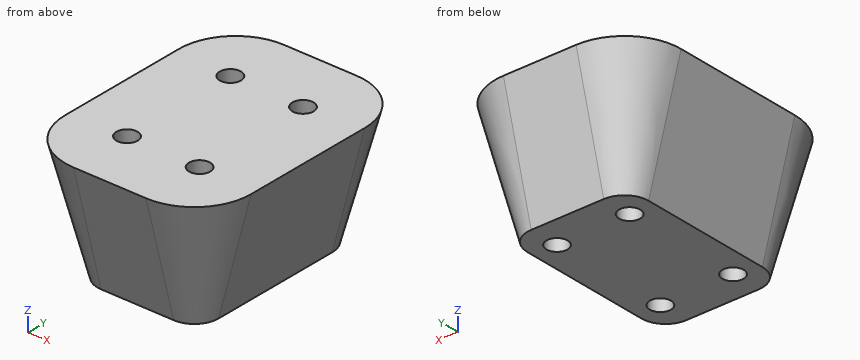
from build123d import *

# Parameters (mm, degrees)
SKETCH1_R           = 1.75
BOSS_EXTRUDE1_DEPTH = 5
BOSS_EXTRUDE2_DEPTH = 20
BOSS_EXTRUDE2_DRAFT = -15
CUT_EXTRUDE1_REACH  = 37.713
SKETCH5_R           = 1.75
CUT_EXTRUDE2_DEPTH  = 5


with BuildPart() as part:
    # Sketch1 → Boss-Extrude1 (new body)
    with BuildSketch(Plane.XY):
        with BuildLine():
            Line((-6, 15), (6, 15))
            ThreePointArc((6, 15), (8.828427125, 13.828427125), (10, 11))
            Line((10, 11), (10, -11))
            ThreePointArc((10, -11), (8.828427125, -13.828427125), (6, -15))
            Line((6, -15), (-6, -15))
            ThreePointArc((-6, -15), (-8.828427125, -13.828427125), (-10, -11))
            Line((-10, -11), (-10, 11))
            ThreePointArc((-10, 11), (-8.828427125, 13.828427125), (-6, 15))
        make_face()
        with Locations((-6, 10)):
            Circle(SKETCH1_R, mode=Mode.SUBTRACT)
        with Locations((6, 10)):
            Circle(SKETCH1_R, mode=Mode.SUBTRACT)
        with Locations((-6, -10)):
            Circle(SKETCH1_R, mode=Mode.SUBTRACT)
        with Locations((6, -10)):
            Circle(SKETCH1_R, mode=Mode.SUBTRACT)
    extrude(amount=BOSS_EXTRUDE1_DEPTH)


with BuildPart() as boss_extrude2_tool:
    # Sketch4 → Boss-Extrude2 (with draft: the straight prism first)
    with BuildSketch(Plane.XY.offset(5)):
        with BuildLine():
            Line((-6, -15), (6, -15))
            ThreePointArc((6, -15), (8.828427125, -13.828427125), (10, -11))
            Line((10, -11), (10, 11))
            ThreePointArc((10, 11), (8.828427125, 13.828427125), (6, 15))
            Line((6, 15), (-6, 15))
            ThreePointArc((-6, 15), (-8.828427125, 13.828427125), (-10, 11))
            Line((-10, 11), (-10, -11))
            ThreePointArc((-10, -11), (-8.828427125, -13.828427125), (-6, -15))
        make_face()
    extrude(amount=BOSS_EXTRUDE2_DEPTH)
    # Boss-Extrude2: the draft: its side faces are tilted about the plane it starts from
    boss_extrude2_sides = [boss_extrude2_tool.faces().sort_by_distance(p)[0] for p in [
        (-10, 0, 15),
        (-8.828427125, -13.828427125, 15),
        (0, -15, 15),
        (8.828427125, -13.828427125, 15),
        (10, 0, 15),
        (8.828427125, 13.828427125, 15),
        (0, 15, 15),
        (-8.828427125, 13.828427125, 15),
    ]]
    draft(boss_extrude2_sides, Plane.XY.offset(5), BOSS_EXTRUDE2_DRAFT)


with BuildPart() as part_1:
    add(part.part)

    # Boss-Extrude2: add boss_extrude2_tool
    add(boss_extrude2_tool.part)

    # Sketch5 → Cut-Extrude1 (cut, up to next)
    with BuildSketch(Plane(origin=(0, 0, 0), x_dir=(-1, 0, 0), z_dir=(0, 0, -1)), mode=Mode.PRIVATE) as cut_extrude1_sk1:
        with Locations(Location((-6, -10, 0), (0, 0, 180))):
            Circle(SKETCH5_R)
    cut_extrude1_tool1 = extrude(cut_extrude1_sk1.sketch, amount=-CUT_EXTRUDE1_REACH, mode=Mode.PRIVATE) & part_1.part
    # Sketch5 → Cut-Extrude1 (cut, up to next)
    with BuildSketch(Plane(origin=(0, 0, 0), x_dir=(-1, 0, 0), z_dir=(0, 0, -1)), mode=Mode.PRIVATE) as cut_extrude1_sk2:
        with Locations(Location((6, -10, 0), (0, 0, 180))):
            Circle(SKETCH5_R)
    cut_extrude1_tool2 = extrude(cut_extrude1_sk2.sketch, amount=-CUT_EXTRUDE1_REACH, mode=Mode.PRIVATE) & part_1.part
    # Sketch5 → Cut-Extrude1 (cut, up to next)
    with BuildSketch(Plane(origin=(0, 0, 0), x_dir=(-1, 0, 0), z_dir=(0, 0, -1)), mode=Mode.PRIVATE) as cut_extrude1_sk3:
        with Locations(Location((6, 10, 0), (0, 0, 180))):
            Circle(SKETCH5_R)
    cut_extrude1_tool3 = extrude(cut_extrude1_sk3.sketch, amount=-CUT_EXTRUDE1_REACH, mode=Mode.PRIVATE) & part_1.part
    # Sketch5 → Cut-Extrude1 (cut, up to next)
    with BuildSketch(Plane(origin=(0, 0, 0), x_dir=(-1, 0, 0), z_dir=(0, 0, -1)), mode=Mode.PRIVATE) as cut_extrude1_sk4:
        with Locations(Location((-6, 10, 0), (0, 0, 180))):
            Circle(SKETCH5_R)
    cut_extrude1_tool4 = extrude(cut_extrude1_sk4.sketch, amount=-CUT_EXTRUDE1_REACH, mode=Mode.PRIVATE) & part_1.part
    add(cut_extrude1_tool1.solids().sort_by_distance((6, -10, 0))[0], mode=Mode.SUBTRACT)
    add(cut_extrude1_tool2.solids().sort_by_distance((-6, -10, 0))[0], mode=Mode.SUBTRACT)
    add(cut_extrude1_tool3.solids().sort_by_distance((-6, 10, 0))[0], mode=Mode.SUBTRACT)
    add(cut_extrude1_tool4.solids().sort_by_distance((6, 10, 0))[0], mode=Mode.SUBTRACT)

    # Sketch6 → Cut-Extrude2 (cut)
    with BuildSketch(Plane(origin=(0, 0, 0), x_dir=(-1, 0, 0), z_dir=(0, 0, -1))):
        with BuildLine():
            Line((6, -15), (-6, -15))
            ThreePointArc((-6, -15), (-8.828427125, -13.828427125), (-10, -11))
            Line((-10, -11), (-10, 11))
            ThreePointArc((-10, 11), (-8.828427125, 13.828427125), (-6, 15))
            Line((-6, 15), (6, 15))
            ThreePointArc((6, 15), (8.828427125, 13.828427125), (10, 11))
            Line((10, 11), (10, -11))
            ThreePointArc((10, -11), (8.828427125, -13.828427125), (6, -15))
        make_face()
    extrude(amount=-CUT_EXTRUDE2_DEPTH, mode=Mode.SUBTRACT)


solid = part_1.part
For this review, take the finished solid that the model builds, in its own axes (mm). Round coordinates to 2 decimals unless told otherwise and drop trailing zeros. Order: outer loops, then holes, each group sorted by start corner. A loop starts at its lowest first (then second) coordinate and runs counter-clockwise, first axis right, second up. Notation, with made-up numbers: (16.5, 60) -> (34.5, 60) arc R12 ccw to (34.5, 71) -> close; hole circle Ø5 at (83, -34). An arc over 180 degrees is marked (long way). Put each result on its own line as item: value.
Q1. Insertion check: pin 1 Ø4.5 at (x, y) = (6, 10) entering from +Z; pin 2 Ø12 at (x, z) = (1.5, 11) entering from +Y; pin 3 Ø6 at (y, z) = (13, 7.5) entering from +X; pin 4 Ø3 at (x, y) = (-6, -10) entering from -Z. Each pin has a flat end and moves straight along its axis. Give the tip position at first contact, or say it passes through.
Check result:
pin 1: z = 25
pin 2: y = 18.22
pin 3: x = 11.35
pin 4: through
Q2. Add section B-B on x = 2. Write out the cut boundary in (y, z).
Check result:
outline: (-20.36, 25) -> (-15, 5) -> (15, 5) -> (20.36, 25) -> close
Q3. Add section A-A on y = -10. Write out the cut boundary in (x, z).
Check result:
outline: (-15.36, 25) -> (-10, 5) -> (-7.75, 5) -> (-7.75, 25) -> close; (-4.25, 5) -> (4.25, 5) -> (4.25, 25) -> (-4.25, 25) -> close; (7.75, 5) -> (10, 5) -> (15.36, 25) -> (7.75, 25) -> close
Q4. Add section C-C on z = 8.5. Write out the cut boundary in (x, y), plus the area to 3 significant figures.
Check result:
outline: (-10.94, -11) arc R4.94 ccw to (-6, -15.94) -> (6, -15.94) arc R4.94 ccw to (10.94, -11) -> (10.94, 11) arc R4.94 ccw to (6, 15.94) -> (-6, 15.94) arc R4.94 ccw to (-10.94, 11) -> close; hole circle Ø3.5 at (-6, -10); hole circle Ø3.5 at (-6, 10); hole circle Ø3.5 at (6, -10); hole circle Ø3.5 at (6, 10)
area: 638 mm2
Q5. For probe 1 along X at (y, z) = (10, 12.25); probe 2 along Y at (x, z) = (6, 17.5); probe 3 along Y at (x, z) = (6, 13.5), list the stretches that pass through material, from the lowest coordinate up. Write a range as [from, to].
Check result:
probe 1: [-11.94, -7.75], [-4.25, 4.25], [7.75, 11.94]
probe 2: [-18.35, -11.75], [-8.25, 8.25], [11.75, 18.35]
probe 3: [-17.28, -11.75], [-8.25, 8.25], [11.75, 17.28]
Q6. Add section D-D on y = 2.5. Write out the cut boundary in (x, z), plus the area to 3 significant figures.
Check result:
outline: (-15.36, 25) -> (-10, 5) -> (10, 5) -> (15.36, 25) -> close
area: 507 mm2
